from build123d import *

# Parameters (mm, degrees)
SKETCH1_W           = 200
SKETCH1_H           = 155
BOSS_EXTRUDE1_DEPTH = 3
SKETCH2_R           = 2.05
CUT_EXTRUDE1_DEPTH  = 4
FILLET1_R           = 10
SKETCH6_R           = 2.05
SKETCH6_W           = 13
SKETCH6_H           = 25.5
CUT_EXTRUDE2_DEPTH  = 4


with BuildPart() as part:
    # Sketch1 → Boss-Extrude1 (new body)
    with BuildSketch(Plane(origin=(0, 0, 0), x_dir=(1, 0, 0), z_dir=(0, 1, 0))):
        with Locations((100, 77.5)):
            Rectangle(SKETCH1_W, SKETCH1_H)
    extrude(amount=BOSS_EXTRUDE1_DEPTH)

    # Sketch2 → Cut-Extrude1 (cut, through all)
    with BuildSketch(Plane(origin=(0, 3, 0), x_dir=(1, 0, 0), z_dir=(0, 1, 0))):
        with Locations((37.5, 7.95)):
            Circle(SKETCH2_R)
        with Locations((67.5, 7.95)):
            Circle(SKETCH2_R)
        with Locations((132.5, 7.95)):
            Circle(SKETCH2_R)
        with Locations((162.5, 7.95)):
            Circle(SKETCH2_R)
        with Locations((162.5, 147.05)):
            Circle(SKETCH2_R)
        with Locations((132.5, 147.05)):
            Circle(SKETCH2_R)
        with Locations((67.5, 147.05)):
            Circle(SKETCH2_R)
        with Locations((37.5, 147.05)):
            Circle(SKETCH2_R)
    extrude(amount=-CUT_EXTRUDE1_DEPTH, mode=Mode.SUBTRACT)

    # Fillet1
    fillet1_edges = [part.edges().sort_by_distance(p)[0] for p in [
        (0, 1.5, -155),
        (200, 1.5, -155),
        (200, 1.5, 0),
        (0, 1.5, 0),
    ]]
    fillet(fillet1_edges, radius=FILLET1_R)

    # Sketch6 → Cut-Extrude2 (cut, through all)
    with BuildSketch(Plane(origin=(0, 3, 0), x_dir=(1, 0, 0), z_dir=(0, 1, 0))):
        with Locations((10.05, 143.95)):
            Circle(SKETCH6_R)
        with Locations((21.15, 118.2)):
            Circle(SKETCH6_R)
        with Locations((36.95, 122.6)):
            Circle(SKETCH6_R)
        with Locations((43.95, 127.3)):
            Circle(SKETCH6_R)
        with Locations((43.95, 27.7)):
            Circle(SKETCH6_R)
        with Locations((36.95, 32.4)):
            Circle(SKETCH6_R)
        with Locations((10.05, 11.05)):
            Circle(SKETCH6_R)
        with Locations((21.15, 36.8)):
            Circle(SKETCH6_R)
        with Locations((189.95, 143.95)):
            Circle(SKETCH6_R)
        with Locations((110.45, 146.45)):
            Circle(SKETCH6_R)
        with Locations((189.95, 11.05)):
            Circle(SKETCH6_R)
        with Locations((110.45, 8.55)):
            Circle(SKETCH6_R)
        with BuildLine():
            Line((12.1, 118.2), (12.1, 36.8))
            ThreePointArc((12.1, 36.8), (10.05, 34.75), (8, 36.8))
            Line((8, 36.8), (8, 118.2))
            ThreePointArc((8, 118.2), (10.05, 120.25), (12.1, 118.2))
        make_face()
        with Locations((23.85, 77.5)):
            Rectangle(SKETCH6_W, SKETCH6_H)
    extrude(amount=-CUT_EXTRUDE2_DEPTH, mode=Mode.SUBTRACT)


solid = part.part
Read the model definition and answer for the solid it produces. Units are mm, in the model's axes. Round coordinates to 2 decimals unless told otherwise and drop trailing zeros. Loops run counter-clockwise (first coordinate to the right, second up) from the corner with the lowest first, then second, coordinate; pieces in that order, holes last.
Q1. This flat-tipped pin is pushed along its axis until it touches: pin 1 (2.5 mm diameter, centred on x = 132.5, z = -7.95, fed in from -Y). Where does it stop, or does it pass through?
Q2. Section C-C on y = 2.3 is taken. Give the number of separate pieces and of enclosed holes in the cut face, and give its area (3 significant figures).
Q3. Consider probe 1 along Z at (x, y) = (110, 1.8); probe 2 along X at (y, z) = (0.2, -75.5); probe 3 along X at (y, z) = (2.05, -36.8). Determine where each line is inside the solid, lowest interval first.
Q4. Section A-A on z = -82 is taken. Write down the section's boundary in (x, y), and give its area (3 significant figures).
Q5. Section B-B on z = -122.6 is taken. Write down the section's boundary in (x, y), and give its area (3 significant figures).
Q6. Determine the mould class of faces 1 (the face through (108.4, 1.5, -8.6)), 2 (the face through (99, 3, -79)), 3 (the face through (196.99, 1.52, -2.85)) for opening direction Z: released by +Z, released by -Z, zero draft, split by the parting line, or undercut.
Output:
1. pin 1: passes through
2. separate pieces: 1
2. enclosed holes: 22
2. area: 30,000 mm2
3. probe 1: z = -155 to -148.45, -144.45 to -10.55, -6.55 to 0
3. probe 2: x = 0 to 8, 12.1 to 17.35, 30.35 to 200
3. probe 3: x = 0 to 8, 12.1 to 19.1, 23.2 to 200
4. outline: (0, 0) - (8, 0) - (8, 3) - (0, 3) - close; (12.1, 0) - (17.35, 0) - (17.35, 3) - (12.1, 3) - close; (30.35, 0) - (200, 0) - (200, 3) - (30.35, 3) - close
4. area: 549 mm2
5. outline: (0, 0) - (34.9, 0) - (34.9, 3) - (0, 3) - close; (39, 0) - (200, 0) - (200, 3) - (39, 3) - close
5. area: 588 mm2
6. face 1: undercut
6. face 2: zero draft
6. face 3: released by +Z
